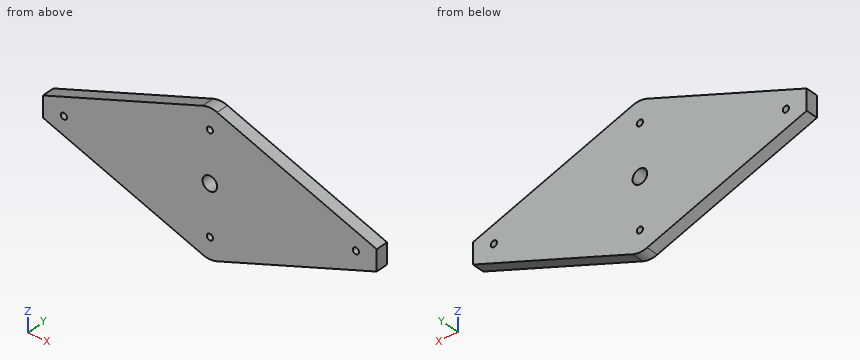
from build123d import *

# Parameters (mm, degrees)
SKETCH1_R      = 0.75
SKETCH1_R_2    = 1.75
EXTRUDE1_DEPTH = 1.5


with BuildPart() as part:
    # Sketch1 → Extrude1 (new body, symmetric)
    with BuildSketch(Plane(origin=(0, 0, 0), x_dir=(1, 0, 0), z_dir=(0, 1, 0))):
        with BuildLine():
            Line((-1.738414467, 16.688060915), (-40, 2.5))
            Line((-40, 2.5), (-40, -2.5))
            Line((-40, -2.5), (-1.738414467, -16.688060915))
            ThreePointArc((-1.738414467, -16.688060915), (0, -17), (1.738414467, -16.688060915))
            Line((1.738414467, -16.688060915), (40, -2.5))
            Line((40, -2.5), (40, 2.5))
            Line((40, 2.5), (1.738414467, 16.688060915))
            ThreePointArc((1.738414467, 16.688060915), (0, 17), (-1.738414467, 16.688060915))
        make_face()
        with Locations(Location((0, 12, 0), (0, 0, 270))):  # turned: the seam where the file's is
            Circle(SKETCH1_R, mode=Mode.SUBTRACT)
        with Locations(Location((0, -12, 0), (0, 0, 270))):  # turned: the seam where the file's is
            Circle(SKETCH1_R, mode=Mode.SUBTRACT)
        with Locations(Location((35, 0, 0), (0, 0, 270))):  # turned: the seam where the file's is
            Circle(SKETCH1_R, mode=Mode.SUBTRACT)
        with Locations(Location((-35, 0, 0), (0, 0, 270))):  # turned: the seam where the file's is
            Circle(SKETCH1_R, mode=Mode.SUBTRACT)
        with Locations(Location((0, 0, 0), (0, 0, 270))):  # turned: the seam where the file's is
            Circle(SKETCH1_R_2, mode=Mode.SUBTRACT)
    extrude(amount=EXTRUDE1_DEPTH, both=True)


solid = part.part
Verification items for the finished model (mm, model axes). Give positions to 0.01 mm unless a question says otherwise; leave off trailing zeros. Order: outer loops, then holes, each group sorted by start corner. A loop starts at its lowest first (then second) coordinate and runs counter-clockwise, first axis right, second up. Notation, with made-up numbers: M 66.5,29.25 L 108.5,29.25 A25 ccw 108.5,62.25 Z; hole C 87.25,-36.5 d9. An arc over 180 degrees is marked long. Answer as a JSON object with one key per item and string values. Group by question number.
1) Cross-section at A-A (z = 0). Enter the section's corners in (x, y).
2) Scan lines: line 1 along X through (y, z) = (-0.05, 0); line 2 along X through (y, z) = (0.2, 1); line 3 along Z through (x, y) = (35, 0.75). Record each from-to range of solid material in increasing order. Write a range as [from, to].
3) Cross-section at B-B (x = 0). Enter the section's corners in (y, z), then the cut area to 3 significant figures.
4) Cross-section at C-C (x = -35). Enter the section's corners in (y, z), then the cut area to 3 significant figures.
5) Depth check by flat-ended pin: pin 1 Ø0.9 at (x, z) = (-35, 0) entering from -Y. Enter the tip coordinate at first touch or a pass-through.
6) Cross-section at D-D (y = -0.7). Enter the section's corners in (x, z), then the cut area to 3 significant figures.
Result sheet:
{
 "1": {"outline": "M -40,-1.5 L -35.75,-1.5 L -35.75,1.5 L -40,1.5 Z; M -34.25,-1.5 L -1.75,-1.5 L -1.75,1.5 L -34.25,1.5 Z; M 1.75,-1.5 L 34.25,-1.5 L 34.25,1.5 L 1.75,1.5 Z; M 35.75,-1.5 L 40,-1.5 L 40,1.5 L 35.75,1.5 Z"},
 "2": {"line 1": "x = [-40, -35.75], [-34.25, -1.75], [1.75, 34.25], [35.75, 40]", "line 2": "x = [-40, -1.44], [1.44, 40]", "line 3": "z = [-4.35, -0.75], [0.75, 4.35]"},
 "3": {"outline": "M -1.5,-17 L 1.5,-17 L 1.5,-12.75 L -1.5,-12.75 Z; M -1.5,-11.25 L 1.5,-11.25 L 1.5,-1.75 L -1.5,-1.75 Z; M -1.5,1.75 L 1.5,1.75 L 1.5,11.25 L -1.5,11.25 Z; M -1.5,12.75 L 1.5,12.75 L 1.5,17 L -1.5,17 Z", "area": "82.5 mm2"},
 "4": {"outline": "M -1.5,-4.35 L 1.5,-4.35 L 1.5,-0.75 L -1.5,-0.75 Z; M -1.5,0.75 L 1.5,0.75 L 1.5,4.35 L -1.5,4.35 Z", "area": "21.6 mm2"},
 "5": {"pin 1": "passes through"},
 "6": {"outline": "M -40,-2.5 L -1.74,-16.69 A5 ccw 1.74,-16.69 L 40,-2.5 L 40,2.5 L 1.74,16.69 A5 ccw -1.74,16.69 L -40,2.5 Z; hole C -35,0 d1.5; hole C 0,0 d3.5; hole C 0,-12 d1.5; hole C 0,12 d1.5; hole C 35,0 d1.5", "area": "1,570 mm2"}
}
